from build123d import *

# Parameters (mm, degrees)
SKETCH4_W               = 41.275
SKETCH4_H               = 41.275
SKETCH4_R               = 2.286
SKETCH4_R_2             = 6.35
BOSS_EXTRUDE1_DEPTH     = 12.7
SKETCH6_R               = 10.922
SKETCH6_R_2             = 6.35
BOSS_EXTRUDE2_DEPTH     = 9.525
CUT_EXTRUDE1_DEPTH      = 23.225
CHAMFER1_SIZE           = 1.27
CHAMFER1_SIZE2          = 0.56544043
CHAMFER3_SIZE           = 0.635
SKETCH18_R              = 2.1463
CUT_EXTRUDE2_DEPTH      = 18.847032
CUT_EXTRUDE2_DEPTH_BACK = 2.54
SKETCH19_R              = 3.81
CUT_EXTRUDE3_DEPTH      = 4.1656
CUT_EXTRUDE3_DEPTH_BACK = 13.484099492
CUT_EXTRUDE4_DEPTH      = 1.24968
CHAMFER4_SIZE           = 0.381
CHAMFER4_SIZE2          = 0.169632129
FILLET1_R               = 0.381
FILLET2_R               = 2.921


with BuildPart() as part:
    # Sketch4 → Boss-Extrude1 (new body)
    with BuildSketch(Plane.XY):
        Rectangle(SKETCH4_W, SKETCH4_H)
        with Locations((-15.875, -15.875)):
            Circle(SKETCH4_R, mode=Mode.SUBTRACT)
        with Locations((15.875, -15.875)):
            Circle(SKETCH4_R, mode=Mode.SUBTRACT)
        with Locations((15.875, 15.875)):
            Circle(SKETCH4_R, mode=Mode.SUBTRACT)
        with Locations((-15.875, 15.875)):
            Circle(SKETCH4_R, mode=Mode.SUBTRACT)
        Circle(SKETCH4_R_2, mode=Mode.SUBTRACT)
    extrude(amount=-BOSS_EXTRUDE1_DEPTH)

    # Sketch6 → Boss-Extrude2 (add)
    with BuildSketch(Plane.XY):
        Circle(SKETCH6_R)
        Circle(SKETCH6_R_2, mode=Mode.SUBTRACT)
    extrude(amount=BOSS_EXTRUDE2_DEPTH)

    # Sketch8 → Cut-Extrude1 (cut, through all)
    with BuildSketch(Plane.XY.offset(9.525)):
        with BuildLine():
            Line((11.388684671, -21.43125), (2.415183293, -5.88868969))
            ThreePointArc((2.415183293, -5.88868969), (2.996248621, -3.720124362), (5.16481395, -4.30118969))
            Line((5.16481395, -4.30118969), (14.138315329, -19.84375))
            ThreePointArc((14.138315329, -19.84375), (13.55725, -22.012315329), (11.388684671, -21.43125))
        make_face()
    extrude(amount=-CUT_EXTRUDE1_DEPTH, mode=Mode.SUBTRACT)

    # Chamfer1
    chamfer1_edges = [part.edges().sort_by_distance(p)[0] for p in [
        (-6.09154739, 9.065491404, 9.525),
    ]]
    chamfer1_side = [part.faces().sort_by_distance(p)[0] for p in [
        (-6.09154739, 9.065491404, 4.7625),
    ]]
    chamfer(chamfer1_edges, length=CHAMFER1_SIZE, length2=CHAMFER1_SIZE2, reference=chamfer1_side[0])

    # Chamfer3
    chamfer3_edges = [part.edges().sort_by_distance(p)[0] for p in [
        (0, 20.6375, -12.7),
        (-20.6375, 0, -12.7),
        (-4.853543552, -20.6375, -12.7),
        (-20.6375, 0, 0),
        (17.49425, -20.6375, -12.7),
        (0, 20.6375, 0),
        (17.49425, -20.6375, 0),
        (20.6375, 0, 0),
        (-4.853543552, -20.6375, 0),
        (20.6375, 0, -12.7),
        (-20.6375, -20.6375, -6.35),
        (-20.6375, 20.6375, -6.35),
        (20.6375, 20.6375, -6.35),
        (20.6375, -20.6375, -6.35),
    ]]
    chamfer(chamfer3_edges, length=CHAMFER3_SIZE)

    # Sketch18 → Cut-Extrude2 (cut, two sides)
    with BuildSketch(Plane(origin=(13.602877332, 7.853624889, 0), x_dir=(0, 0, -1), z_dir=(-0.866025404, -0.5, 0))) as cut_extrude2_sk:
        with Locations((6.35, 14.069245336)):
            Circle(SKETCH18_R)
    extrude(amount=CUT_EXTRUDE2_DEPTH, mode=Mode.SUBTRACT)
    extrude(cut_extrude2_sk.sketch, amount=-CUT_EXTRUDE2_DEPTH_BACK, mode=Mode.SUBTRACT)

    # Sketch19 → Cut-Extrude3 (cut, two sides)
    with BuildSketch(Plane(origin=(13.602877332, 7.853624889, 0), x_dir=(0, 0, -1), z_dir=(-0.866025404, -0.5, 0))) as cut_extrude3_sk:
        with Locations((6.35, 14.069245336)):
            Circle(SKETCH19_R)
    extrude(amount=CUT_EXTRUDE3_DEPTH, mode=Mode.SUBTRACT)
    extrude(cut_extrude3_sk.sketch, amount=-CUT_EXTRUDE3_DEPTH_BACK, mode=Mode.SUBTRACT)

    # Sketch21 → Revolve2 (revolve)
    with BuildSketch(Plane(origin=(7.034622668, -12.184323873, 0), x_dir=(-0.866025404, -0.5, 0), z_dir=(0.5, -0.866025404, 0))):
        Polygon((-15.707249779, 6.35), (7.878464507, 6.35), (7.878464507, 8.4328), (-11.922649779, 8.4328), (-11.922649779, 9.779), (-15.707249779, 9.779), align=None)
    revolve(axis=Axis((20.6375, -4.330698984, -6.35), (-0.866025404, -0.5, 0)))

    # Sketch22 → Cut-Extrude4 (cut)
    with BuildSketch(Plane(origin=(13.602877332, 7.853624889, 0), x_dir=(0, 0, -1), z_dir=(0.866025404, 0.5, 0))):
        Polygon((6.35, -16.131468329), (8.1359375, -15.100356833), (8.1359375, -13.03813384), (6.35, -12.007022344), (4.5640625, -13.03813384), (4.5640625, -15.100356833), align=None)
    extrude(amount=-CUT_EXTRUDE4_DEPTH, mode=Mode.SUBTRACT)

    # Chamfer4
    chamfer4_edges = [part.edges().sort_by_distance(p)[0] for p in [
        (20.6375, -4.330698984, -2.921),
    ]]
    chamfer4_side = [part.faces().sort_by_distance(p)[0] for p in [
        (18.998720128, -5.276848984, -2.921),
    ]]
    chamfer(chamfer4_edges, length=CHAMFER4_SIZE, length2=CHAMFER4_SIZE2, reference=chamfer4_side[0])

    # Fillet1
    fillet1_edges = [part.edges().sort_by_distance(p)[0] for p in [
        (20.6375, -8.730108035, -6.35000004),
        (20.6375, 0.068710067, -6.34999996),
    ]]
    fillet(fillet1_edges, radius=FILLET1_R)

    # Fillet2
    fillet2_edges = [part.edges().sort_by_distance(p)[0] for p in [
        (-6.09154739, 9.065491404, 0),
    ]]
    fillet(fillet2_edges, radius=FILLET2_R)


solid = part.part
Source: CAD feature listing. Evaluate the final solid. Frame: model axes, mm. A direction names the side the tool comes from. Give positions to 0.01 mm unless a question says otherwise; leave off trailing zeros. Write each loop counter-clockwise with the first axis right and the second up, starting at its lowest first coordinate (ties: lowest second). Pieces come first, ordered by that corner, then holes. Notation, with made-up numbers: (82, 20.25) - (95, 20.25) arc R19 ccw to (95, 38.25) - close; hole circle Ø4 at (41, -0.75). An arc over 180 degrees is marked (long way). Write item = value, one per line. Start each with the question number.
Q1. Material intervals for probe 1 along X at (y, z) = (-3, -8); probe 2 along Z at (x, y) = (-8.5, -13); probe 3 along Y at (x, z) = (0, -5), sorted ascending.
Q2. Reachability of faces 1 (the flat face through (20, -5, -8.136)), 2 (the flat face through (-5, 14, 0)), 3 (the flat face through (20.66, -4.37, -8.48)), 4 (the cylindrical face through (17.987, 14.999, -6.261)) from +Z, -Z, +X, -X, +Y, -Y: full face, straight path, thin tool, end or side. Return the list, or none.
Q3. Cut plane B-B, the plane z = -1.5. Give the number of separate pieces and of enclosed holes in the cut face, then the cut area to 3 significant figures.
Q4. Draft query along Z for faces 5 (the flat face through (20.881, -5.984, -7.23)), 6 (the flat face through (4.5, 4.7, 9.525)), 7 (the cylindrical face through (-14.82, -17.903, -6.261)). Return one class per face: +Z half, -Z half, draft (parallel to the pull), parting line (faces both ways), or undercut.
Q5. Pin query (flat end, axial travel): pin 1 Ø1.7 at (x, y) = (19.5, -4) entering from +Z; pin 2 Ø6 at (y, z) = (12.5, 2.5) entering from -X. Return the tip coordinate at first contact, or that it passes through.
Q6. Cut plane C-C, the plane x = -16. Return loops of the section in (y, z) (1 decimal), then the cut area to 3 significant figures.
Computed values:
q1.probe_1 = -20.64 to -5.6, 5.6 to 16.07, 16.93 to 19.87
q1.probe_2 = -12.7 to 0
q1.probe_3 = -20.64 to -6.35, 6.35 to 20.64
q2.face_1 = none
q2.face_2 = +Z
q2.face_3 = +X
q2.face_4 = +Z, -Z
q3.separate_pieces = 1
q3.enclosed_holes = 4
q3.area = 1,450 mm²
q4.face_5 = undercut
q4.face_6 = +Z half
q4.face_7 = draft
q5.pin_1 = 0
q5.pin_2 = -20.5
q6.outline = (-20.6, -12.1) - (-20, -12.7) - (-18.2, -12.7) - (-18.2, 0) - (-20, 0) - (-20.6, -0.6) - close; (-13.6, -12.7) - (13.6, -12.7) - (13.6, 0) - (-13.6, 0) - close; (18.2, -12.7) - (20, -12.7) - (20.6, -12.1) - (20.6, -0.6) - (20, 0) - (18.2, 0) - close
q6.area = 407 mm²
